Could you check a few things on this drawing? It's one solid part, dimensions in mm from its lowest x, y, z. A direction names the side the tool comes from. Give positions to 0.01 mm unless a question says otherwise; leave off trailing zeros. Order: outer loops, then holes, each group sorted by start corner. A loop starts at its lowest first (then second) coordinate and runs counter-clockwise, first axis right, second up. Notation, with made-up numbers: (-16, -29) - (13, -29) arc R9 cw to (13, -21) - close; hole circle Ø11 at (-26.5, -0.75). An arc over 180 degrees is marked (long way). Answer as CSV lines item,"result".
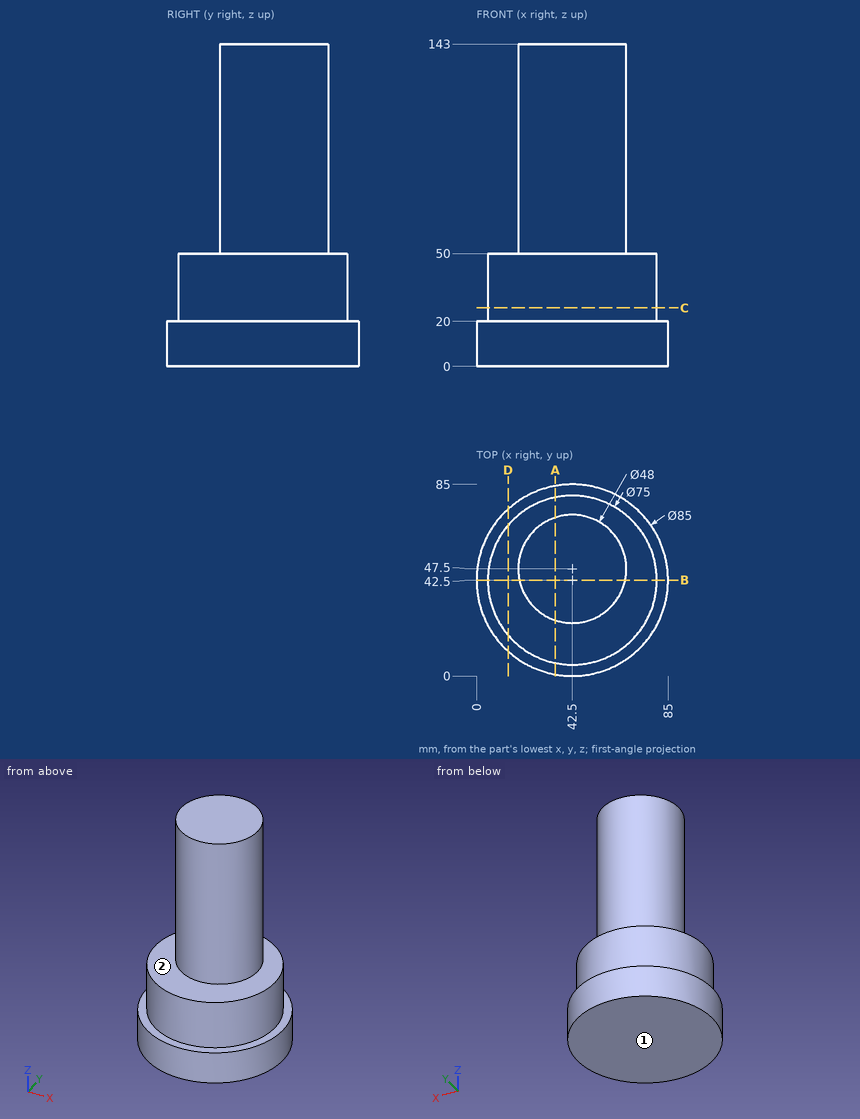
1) I'm going to push flat-ended pins straight in: P1, Ø5, axis at x = 31, z = 110.5, coming from the +Y side; P2, Ø1.5, axis at y = 34, z = 122, coming from the +X side; P3, Ø2, axis at y = 57, z = 66.5, coming from the -X side; P4, Ø4, axis at x = 10.5, y = 27, coming from the -Z side. Where does each tip first touch, or does it pass through?
Answer block:
P1,"y = 69.75"
P2,"x = 62.83"
P3,"x = 20.06"
P4,"z = 0"
2) I need wall thicknesses on line 1 along Z through (x, y) = (26.5, 66.5); line 2 along Z through (x, y) = (61.5, 75.5); line 3 along Y through (x, z) = (42, 97.5). Which ranges of each line are inside material? Lowest first, please. Write a range as [from, to].
Answer block:
line 1,"[0, 50]"
line 2,"[0, 20]"
line 3,"[23.51, 71.49]"
3) Which directions (+Z, -Z, +X, -X, +Y, -Y) give clear straight access to the entire face, cutting with the end or side of a thin tool? Please do the marked faces 1 and 2.
Answer block:
face 1,"-Z, +X, -X, +Y, -Y"
face 2,"+Z"
4) I want a section at B-B on y = 42.5. Write out the boundary of the cut face in (x, z), plus the area to 3 significant figures.
Answer block:
outline,"(0, 0) - (85, 0) - (85, 20) - (80, 20) - (80, 50) - (65.97, 50) - (65.97, 143) - (19.03, 143) - (19.03, 50) - (5, 50) - (5, 20) - (0, 20) - close"
area,"8,320 mm2"
5) I want a section at A-A on x = 35. Write out the boundary of the cut face in (y, z), plus the area to 3 significant figures.
Answer block:
outline,"(0.67, 0) - (84.33, 0) - (84.33, 20) - (79.24, 20) - (79.24, 50) - (70.3, 50) - (70.3, 143) - (24.7, 143) - (24.7, 50) - (5.76, 50) - (5.76, 20) - (0.67, 20) - close"
area,"8,120 mm2"
6) I want a section at C-C on z = 26. Write out the boundary of the cut face in (x, y).
Answer block:
outline,"circle Ø75 at (42.5, 42.5)"
7) I want a section at D-D on x = 14. Write out the boundary of the cut face in (y, z), plus the area to 3 significant figures.
Answer block:
outline,"(10.97, 0) - (74.03, 0) - (74.03, 20) - (66.87, 20) - (66.87, 50) - (18.13, 50) - (18.13, 20) - (10.97, 20) - close"
area,"2,720 mm2"
